Can you work these out from the model? Positions are in its coordinate system, mm. A direction names the side the tool comes from. Give positions to 0.01 mm unless a question says otherwise; leave off trailing zeros. Loops run counter-clockwise (first coordinate to the right, second up) from the corner with the lowest first, then second, coordinate; pieces in that order, holes last. Notation, with made-up numbers: M 57,45.25 L 78,45.25 A31 cw 78,77.25 Z; hole C 45,47 d6. An arc over 180 degrees is marked long. Answer as a JSON object with one key per item and string values.
```python
from build123d import *

# Parameters (mm, degrees)
SKETCH1_R           = 22.5
SKETCH1_R_2         = 12.5
BOSS_EXTRUDE1_DEPTH = 75
SKETCH2_W           = 10
SKETCH2_H           = 19.424824541
CUT_EXTRUDE1_DEPTH  = 50


with BuildPart() as part:
    # Sketch1 → Boss-Extrude1 (new, symmetric)
    with BuildSketch(Plane.XY):
        Circle(SKETCH1_R)
        Circle(SKETCH1_R_2, mode=Mode.SUBTRACT)
    extrude(amount=BOSS_EXTRUDE1_DEPTH, both=True)

    # Sketch2 → Cut-Extrude1 (cut)
    with BuildSketch(Plane.XY.offset(75)):
        with Locations((0, 26.21241227)):
            Rectangle(SKETCH2_W, SKETCH2_H)
    cut_extrude1 = extrude(amount=-CUT_EXTRUDE1_DEPTH, mode=Mode.SUBTRACT)

    # Mirror1: Cut-Extrude1 across plane
    add(cut_extrude1.mirror(Plane.XY), mode=Mode.SUBTRACT)


solid = part.part
```
1) Will these pins go through, and if not, where does the flat tip stop? pin 1 Ø1 at (y, z) = (-14, 13) entering from -X; pin 2 Ø2.5 at (y, z) = (19, 53) entering from +X; pin 3 Ø5 at (x, y) = (0.5, 20.5) entering from +Z; pin 4 Ø8 at (x, y) = (-5, -3.5) entering from -Z.
Answer list:
{"pin 1": "x = -18", "pin 2": "x = 13.83", "pin 3": "z = 25", "pin 4": "through"}
2) Suppose I cut it at D-D, the plane y = -6. Write out the boundary of the cut face in (x, z), and give its area (3 significant figures).
Answer list:
{"outline": "M -21.69,-75 L -10.97,-75 L -10.97,75 L -21.69,75 Z; M 10.97,-75 L 21.69,-75 L 21.69,75 L 10.97,75 Z", "area": "3,220 mm^2"}
3) Suppose I cut it at C-C, the plane z = 50. Write out the boundary of the cut face in (x, y).
Answer list:
{"outline": "M -5,16.5 L -5,21.94 A22.5 ccw long 5,21.94 L 5,16.5 Z; hole C 0,0 d25"}
4) If we mould it in two halves opening along X, with no side actions, what happens to faces 1 (the flat face through (10, -10, -75)), 2 (the cylindrical face through (10.382, -19.961, 1.05)), 3 (the flat face through (5, 19, 50)), 4 (the flat face through (0, 16.5, 50))? For each: +X half, -X half, draft (parallel to the pull), parting line (faces both ways), or undercut.
Answer list:
{"face 1": "draft", "face 2": "parting line", "face 3": "undercut", "face 4": "undercut"}
5) Suppose I cut it at A-A, the plane x = 0. Write out the boundary of the cut face in (y, z), and give its area (3 significant figures).
Answer list:
{"outline": "M -22.5,-75 L -12.5,-75 L -12.5,75 L -22.5,75 Z; M 12.5,-75 L 16.5,-75 L 16.5,-25 L 22.5,-25 L 22.5,25 L 16.5,25 L 16.5,75 L 12.5,75 Z", "area": "2,400 mm^2"}
6) Please list where these lines run through material, in increasing order: line 1 along Y through (x, z) = (0, 13); line 2 along Y through (x, z) = (0, 26); line 3 along X through (y, z) = (18, -44). Write a range as from..to.
Answer list:
{"line 1": "-22.5..-12.5, 12.5..22.5", "line 2": "-22.5..-12.5, 12.5..16.5", "line 3": "-13.5..-5, 5..13.5"}
7) For faces 5 (the flat face through (-5, 19, 50)), 6 (the flat face through (10, -10, 75)), 7 (the flat face through (0, 16.5, -50)), which set-ups out of +Z, -Z, +X, -X, +Y, -Y let a thin tool reach every point of the face, with its end or its side?
Answer list:
{"face 5": "+Z, +Y", "face 6": "+Z, +X, -X, +Y, -Y", "face 7": "-Z, +Y"}
8) Suppose I cut it at B-B, the plane y = 0. Write out the boundary of the cut face in (x, z), and give its area (3 significant figures).
Answer list:
{"outline": "M -22.5,-75 L -12.5,-75 L -12.5,75 L -22.5,75 Z; M 12.5,-75 L 22.5,-75 L 22.5,75 L 12.5,75 Z", "area": "3,000 mm^2"}
